The model under review builds one solid part; all positions refer to its coordinate system, in mm. A direction names the side the tool comes from. Coordinates: 2 decimals unless noted, no trailing zeros. Loops run counter-clockwise (first coordinate to the right, second up) from the corner with the lowest first, then second, coordinate; pieces in that order, holes last. Notation, with made-up numbers: (24.25, 7.25) -> (28.25, 7.25) arc R28 ccw to (28.25, 46.25) -> close; hole circle Ø1 at (-26, 81.5). An arc over 180 degrees is marked (long way). One line per question, with ' | ' between items. Start each with the question number.
from build123d import *

# Parameters (mm, degrees)
F0_W      = 152.267947793
F0_H      = 151.1743441224
F1_DEPTH  = 101.6
F2_SIZE   = 50.8
F3_SIZE   = 50.79999
F4_SIZE   = 50.8
F5_T      = -2.54
F7_W      = 151.2815654278
F7_H      = 151.7730951309
F8_DEPTH  = 127
F9_T      = -2.54
F10_W     = 35.6509871781
F10_H     = 76.8820419908
F11_DEPTH = 0.0254
F12_DEPTH = 2.54
F13_DEPTH = 2.54


# Not quite as in the source:
# - a fillet or chamfer is up to 0.001 mm smaller than in the source, because OpenCascade refuses the exact size


with BuildPart() as f1:
    # F0 (on Top) → F1 (new body)
    with BuildSketch(Plane.XY):
        with Locations((-0.6233751774, 0.4115886986)):
            Rectangle(F0_W, F0_H)
    extrude(amount=F1_DEPTH)

    # F2
    f2_edges = [f1.edges().sort_by_distance(p)[0] for p in [
        (-76.757349, 0.411589, 101.6),
        (-0.623375, -75.175583, 101.6),
        (75.510599, 0.411589, 101.6),
        (-0.623375, 75.998761, 101.6),
    ]]
    chamfer(f2_edges, length=F2_SIZE)

    # F3 (size 50.8 in the source; OpenCascade refuses exactly that, so slightly less here)
    f3_edges = [f1.edges().sort_by_distance(p)[0] for p in [
        (-0.623375, -75.175583, 0),
    ]]
    chamfer(f3_edges, length=F3_SIZE)

    # F4
    f4_edges = [f1.edges().sort_by_distance(p)[0] for p in [
        (75.510599, 75.998761, 25.4),
    ]]
    chamfer(f4_edges, length=F4_SIZE)

    # F5
    f5_openings = [f1.faces().sort_by_distance(p)[0] for p in [
        (-0.623375, 0.411589, 101.6),
    ]]
    offset(amount=F5_T, openings=f5_openings)


with BuildPart() as f8:
    # F7 (on Front) → F8 (new body)
    with BuildSketch(Plane.XZ):
        with Locations((-0.3735423088, -0.9954944253)):
            Rectangle(F7_W, F7_H)
    extrude(amount=F8_DEPTH)

    # F9
    f9_openings = [f8.faces().sort_by_distance(p)[0] for p in [
        (-0.373542, -63.5, 74.891053),
    ]]
    offset(amount=F9_T, openings=f9_openings)

    # F10 (on face) → F11 (join)
    with BuildSketch(Plane.XZ.offset(127)):
        with Locations((-27.7109388262, -38.4410209954)):
            Rectangle(F10_W, F10_H)
    extrude(amount=F11_DEPTH)

    # F12 (cut): a face of the model
    f12_faces = [f8.faces().sort_by_distance(p)[0] for p in [
        (-27.7109388262, -127.0254, -38.4410209954),
    ]]
    extrude(f12_faces, amount=-F12_DEPTH, mode=Mode.SUBTRACT)

    # F13 (cut): a face of the model
    f13_faces = [f8.faces().sort_by_distance(p)[0] for p in [
        (-27.7109388262, -124.4854, -38.4410209954),
    ]]
    extrude(f13_faces, amount=-F13_DEPTH, mode=Mode.SUBTRACT)


solid = f8.part
1) Insertion check: pin 1 Ø8 at (x, z) = (-31, -36) entering from -Y; pin 2 Ø2 at (x, y) = (-35, -126) entering from -Z; pin 3 Ø0.8 at (x, z) = (-31.5, -75.5) entering from -Y. Each pin has a flat end and moves straight along its axis. Give the tip position at first contact, or say it passes through.
2) Consider section B-B, the plane z = 26. Write out the cut boundary in (x, y), plus the area to 3 significant figures.
3) Wall thickness on L1, parallel to Y at x = -12, z = 47.5; L2, parallel to X at y = -89, z = 63; L3, parallel to Z at x = 35, y = -78.5: over which ranges is each line inside the solid? List them lowest first.
4) Consider section D-D, the plane x = -48. Write out the cut boundary in (y, z), plus the area to 3 significant figures.
5) Mouldability with a two-part tool opening along Y and no side actions: class faces 4 (the face through (-1, -63, -76.882)), 5 (the face through (-1, 0, 0)), 6 (the face through (-1, -124.46, 1)) as +Y half, -Y half, draft (parallel to the pull), parting line (faces both ways), or undercut.
6) Consider section A-A, the plane x = -19. Write out the cut boundary in (y, z), plus the area to 3 significant figures.
7) Machinability: for faces 1 (the face through (-9.885, -126, -39)), 2 (the face through (-1, -2.54, 1)), 3 (the face through (-1, -127, 0)), which of the approach directions +Z, -Z, +X, -X, +Y, -Y give a long, thin tool a straight path to every point of the face, cutting with its end or side? Answer none if there is none.
8) Consider section C-C, the plane y = -39.5. Write out the cut boundary in (x, z).
Filled sheet:
1) pin 1: y = -2.54 | pin 2: z = 0 | pin 3: y = -121.95
2) outline: (-76.01, -127) -> (75.27, -127) -> (75.27, 0) -> (-76.01, 0) -> close; hole (-73.47, -124.46) -> (72.73, -124.46) -> (72.73, -2.54) -> (-73.47, -2.54) -> close | area: 1,390 mm^2
3) L1: -127 to -124.46, -2.54 to 0 | L2: -76.01 to -73.47, 72.73 to 75.27 | L3: -76.88 to -74.34
4) outline: (-127, -76.88) -> (0, -76.88) -> (0, 74.89) -> (-2.54, 74.89) -> (-2.54, -74.34) -> (-124.46, -74.34) -> (-124.46, 74.89) -> (-127, 74.89) -> close | area: 1,080 mm^2
5) face 4: draft | face 5: +Y half | face 6: undercut
6) outline: (-127, 0) -> (-124.46, 0) -> (-124.46, 74.89) -> (-127, 74.89) -> close; (-121.95, -76.88) -> (0, -76.88) -> (0, 74.89) -> (-2.54, 74.89) -> (-2.54, -74.34) -> (-121.95, -74.34) -> close | area: 879 mm^2
7) face 1: -Z, -Y | face 2: +Z | face 3: +Z, -Z, +X, -X, -Y
8) outline: (-76.01, -76.88) -> (75.27, -76.88) -> (75.27, 74.89) -> (72.73, 74.89) -> (72.73, -74.34) -> (-73.47, -74.34) -> (-73.47, 74.89) -> (-76.01, 74.89) -> close
